```python
from build123d import *

# Parameters (mm, degrees)
SKETCH_1_R          = 14
SKETCH_1_R_2        = 6
EXTRUDE_1_DEPTH     = 6
SKETCH_2_R          = 1.273771183
CUT_EXTRUDE_1_DEPTH = 21.688160866
CUT_EXTRUDE_2_DEPTH = 21.688160866
CHAMFER_1_SIZE      = 0.6


with BuildPart() as part:
    # 草圖1 → 填料-伸長1 (new body)
    with BuildSketch(Plane.XY):
        Circle(SKETCH_1_R)
        Circle(SKETCH_1_R_2, mode=Mode.SUBTRACT)
    extrude(amount=EXTRUDE_1_DEPTH)

    # 草圖2 → 除料-伸長1 (cut, through all)
    with BuildSketch(Plane.XY.offset(6)):
        with Locations((0, -11)):
            Circle(SKETCH_2_R)
        with Locations((-9.526279442, 5.5)):
            Circle(SKETCH_2_R)
        with Locations((9.526279442, 5.5)):
            Circle(SKETCH_2_R)
    extrude(amount=-CUT_EXTRUDE_1_DEPTH, mode=Mode.SUBTRACT)

    # 草圖3 → 除料-伸長2 (cut, through all)
    with BuildSketch(Plane.XY.offset(6)):
        with BuildLine():
            Line((6, 0), (6, 6))
            Line((6, 6), (9.787707238, 10.010034317))
            ThreePointArc((9.787707238, 10.010034317), (0, 14), (-9.787707238, 10.010034317))
            Line((-9.787707238, 10.010034317), (-6, 6))
            Line((-6, 6), (-6, 0))
            Line((-6, 0), (6, 0))
        make_face()
    extrude(amount=-CUT_EXTRUDE_2_DEPTH, mode=Mode.SUBTRACT)

    # 導角1
    chamfer_1_edges = [part.edges().sort_by_distance(p)[0] for p in [
        (0, -14, 6),
        (0, -14, 0),
    ]]
    chamfer(chamfer_1_edges, length=CHAMFER_1_SIZE)


solid = part.part
```
Could you check a few things on this model? Use its own coordinates, in mm. A direction names the side the tool comes from. Coordinates: 2 decimals unless noted, no trailing zeros. Order: outer loops, then holes, each group sorted by start corner. A loop starts at its lowest first (then second) coordinate and runs counter-clockwise, first axis right, second up. Notation, with made-up numbers: M -40,37.5 L 7,37.5 A15 ccw 7,56.5 Z; hole C 18,57 d8. An arc over 180 degrees is marked long. Use one line per item in the form item = value. Start each with the question number.
1. Suppose I cut it at B-B on z = 2.95. Write out the boundary of the cut face in (x, y).
2. Suppose I cut it at A-A on x = 0. Write out the boundary of the cut face in (y, z), then the cut area to 3 significant figures.
3. We'd pull the mould along Y, two halves only. Please class faces 1 (the flat face through (0, -7, 6)), 2 (the cylindrical face through (-0.276, -12.243, 3.042)), 3 (the conical face through (-0.449, -13.555, 0.162)): +Y half, -Y half, draft (parallel to the pull), parting line (faces both ways), or undercut.
4. For pin 1 (5 mm diameter, centred on x = 2, y = 7.5, fed in from +Z) (3 decimals); pin 2 (3 mm diameter, centred on y = -7, z = 5, fed in from -X); pin 3 (2 mm diameter, centred on y = 1.5, z = 5, fed in from -X); pin 4 (2 mm diameter, centred on x = -10, z = 4, fed in from -Y), each with a flat end and sliding along its axis, tell me the tip position at first contact or that it passes through.
5. On a 3-axis mill with a long thin cutter (end or side, diameter ignored), from which of +Z, -Z, +X, -X, +Y, -Y can I reach the whole of each face in a straight line? I mean faces 4 (the cylindrical face through (-9.692, 6.763, 3.042)), 5 (the flat face through (-7.92, 8.03, 3.04)). Say none if no direction works.
6. Please list where these lines run through material, in increasing order: line 1 (Y direction, x = 0, z = 2.2); line 2 (X direction, y = -3, z = 0.6); line 3 (X direction, y = -10, z = 5.2).
7. Suppose I cut it at C-C on y = 5.5. Count the separate pieces of the cut face and the enclosed holes in it, then the cut area to 3 significant figures.
Geometry says:
q1.outline = M -9.79,10.01 A14 ccw long 9.79,10.01 L 6,6 L 6,0 A6 cw -6,0 L -6,6 Z; hole C -9.53,5.5 d2.55; hole C 0,-11 d2.55; hole C 9.53,5.5 d2.55
q2.outline = M -14,0.6 L -13.4,0 L -12.27,0 L -12.27,6 L -13.4,6 L -14,5.4 Z; M -9.73,0 L -6,0 L -6,6 L -9.73,6 Z
q2.area = 32.4 mm^2
q3.face_1 = draft
q3.face_2 = undercut
q3.face_3 = parting line
q4.pin_1 = through
q4.pin_2 = -12.87
q4.pin_3 = -13.99
q4.pin_4 = -10.72
q5.face_4 = +Z, -Z
q5.face_5 = +Z, -Z, +Y
q6.line_1 = -14 to -12.27, -9.73 to -6
q6.line_2 = -13.67 to -5.2, 5.2 to 13.67
q6.line_3 = -9.8 to -0.79, 0.79 to 9.8
q7.separate_pieces = 4
q7.enclosed_holes = 0
q7.area = 51.1 mm^2
